Verification items for the finished model (mm, model axes). Coordinates: 2 decimals unless noted, no trailing zeros. Order: outer loops, then holes, each group sorted by start corner. A loop starts at its lowest first (then second) coordinate and runs counter-clockwise, first axis right, second up. Notation, with made-up numbers: (41, 67.25) -> (84, 67.25) arc R25 ccw to (84, 93.25) -> close; hole circle Ø5 at (46, -7). An arc over 180 degrees is marked (long way). Write item = value, one per line. Start each with the question number.
1. Cross-section at A-A on x = 0. Record the cut outline in (y, z) (3 decimals).
2. Thickness scan on line 1 along Z through (x, y) = (0, 4.25) (3 decimals); line 2 along Z through (x, y) = (-3, 7.75). Record the ranges inside material, lowest first. Write a range as from..to.
3. Release check for a two-part mould opening along Z. For faces 1 (the flat face through (-14, 13.462, 0)), 2 (the cylindrical face through (-1.5, 6.6, -23.6)), 3 (the cylindrical face through (23.393, 6.637, -0.992)), 4 (the cylindrical face through (4.33, 6.64, -32.99)) record: +Z half, -Z half, draft (parallel to the pull), parting line (faces both ways), or undercut.
4. Cross-section at B-B on z = 0. Record the cut outline in (x, y) (3 decimals).
5. Cross-section at D-D on x = 8. Record the cut outline in (y, z).
6. Go/stop test with flat-tipped pins: P1, Ø19, axis at x = 0, z = 0, coming from the +Y side; P2, Ø10.5, axis at x = -26.543, z = 0, coming from the +Y side; P3, Ø2, axis at x = 9.5, y = 10.5, coming from the +Z side; P4, Ø4, axis at x = 1, y = 5.5, coming from the +Z side. Record where each tip stops, or that it passes through.
7. Cross-section at C-C on z = 25. Record the cut outline in (x, y), plus the area to 3 significant figures.
Autodesk Inventor part; units mm, degrees
ref_plane "YZ Plane" through (0, 0, 0) normal (1, 0, 0) x (0, 1, 0)
ref_plane "XZ Plane" through (0, 0, 0) normal (0, 1, 0) x (-1, 0, 0)
ref_plane "XY Plane" through (0, 0, 0) normal (0, 0, 1) x (1, 0, 0)
sketch "Sketch1" plane through (0, 0, 0) normal (0, 1, 0) x (-1, 0, 0)
  circle A0 centre (0, 0) radius 33.274
  circle A1 centre (0, 0) radius 26.543 construction
  circle A2 centre (0, 26.543) radius 3.302
  circle A3 centre (26.543, 0) radius 3.302
  circle A4 centre (0, -26.543) radius 3.302
  circle A5 centre (-26.543, 0) radius 3.302
  circle A6 centre (0, 0) radius 11.8999
  dimension "d0" = 66.548
  dimension "d1" = 53.086
  dimension "d2" = 6.604
  dimension "d3" = 6.604
  dimension "d4" = 6.604
  dimension "d5" = 6.604
  dimension "d6" = 23.7998
extrude "Extrusion1" add sketch "Sketch1" along normal blind 13.462
thread "Thread1"
properties part number "Flange" material "Polycarbonate, Clear"
Worked out:
q1.outline = (0, -33.274) -> (13.462, -33.274) -> (13.462, -29.845) -> (0, -29.845) -> close; (0, -23.241) -> (13.462, -23.241) -> (13.462, -11.9) -> (0, -11.9) -> close; (0, 11.9) -> (13.462, 11.9) -> (13.462, 23.241) -> (0, 23.241) -> close; (0, 29.845) -> (13.462, 29.845) -> (13.462, 33.274) -> (0, 33.274) -> close
q2.line_1 = -33.274..-29.845, -23.241..-11.9, 11.9..23.241, 29.845..33.274
q2.line_2 = -33.14..-27.92, -25.16..-11.52, 11.52..25.16, 27.92..33.14
q3.face_1 = draft
q3.face_2 = undercut
q3.face_3 = undercut
q3.face_4 = parting line
q4.outline = (-33.274, 0) -> (-29.845, 0) -> (-29.845, 13.462) -> (-33.274, 13.462) -> close; (-23.241, 0) -> (-11.9, 0) -> (-11.9, 13.462) -> (-23.241, 13.462) -> close; (11.9, 0) -> (23.241, 0) -> (23.241, 13.462) -> (11.9, 13.462) -> close; (29.845, 0) -> (33.274, 0) -> (33.274, 13.462) -> (29.845, 13.462) -> close
q5.outline = (0, -32.3) -> (13.46, -32.3) -> (13.46, -8.81) -> (0, -8.81) -> close; (0, 8.81) -> (13.46, 8.81) -> (13.46, 32.3) -> (0, 32.3) -> close
q6.P1 = through
q6.P2 = 13.46
q6.P3 = 32.17
q6.P4 = 33.27
q7.outline = (-21.96, 0) -> (-2.92, 0) -> (-2.92, 13.46) -> (-21.96, 13.46) -> close; (2.92, 0) -> (21.96, 0) -> (21.96, 13.46) -> (2.92, 13.46) -> close
q7.area = 513 mm²
